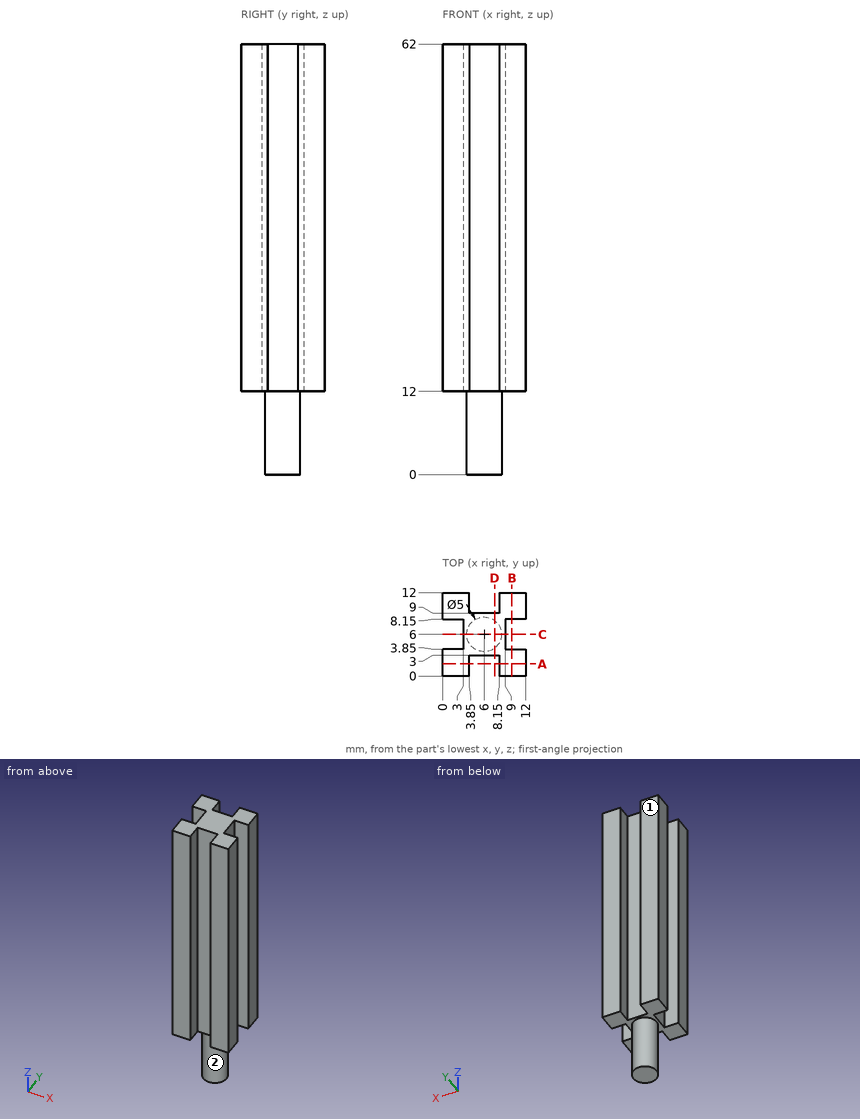
Check sheet for the drawn part. Datum: minimum x, y, z corner. Units: mm. A direction names the side the tool comes from. Round coordinates to 2 decimals unless told otherwise and drop trailing zeros. Order: outer loops, then holes, each group sorted by start corner. A loop starts at its lowest first (then second) coordinate and runs counter-clockwise, first axis right, second up. Notation, with made-up numbers: M 78,-36.75 L 100,-36.75 A20 ccw 100,-21.75 Z; hole C -19.75,9.25 d9. An arc over 180 degrees is marked long. Answer in a Markdown table with one row per item.
(1) Section check D-D on x = 7.5. Record the boundary of the cut face in (y, z), plus the area to 3 significant figures.
Findings:
| item | result |
|---|---|
| outline | M 3,12 L 4,12 L 4,0 L 8,0 L 8,12 L 9,12 L 9,62 L 3,62 Z |
| area | 348 mm^2 |
(2) Material ranges on line 1 along X through (y, z) = (9.75, 57); line 2 along Z through (x, y) = (3.5, 8), recorded low to high. Write a range as from..to.
Findings:
| item | result |
|---|---|
| line 1 | x = 0..3.85, 8.15..12 |
| line 2 | z = 12..62 |
(3) Gauge pin test, flat ends, axial feed: pin 1 (1.3 mm diameter, centred on y = 6, z = 44.5, fed in from -X); pin 2 (1 mm diameter, centred on x = 7, z = 6.5, fed in from +Y); pin 3 (2 mm diameter, centred on x = 5, z = 45.5, fed in from -Y). Record the tip position at first contact, or that the pin passes through.
Findings:
| item | result |
|---|---|
| pin 1 | stops at x = 3 |
| pin 2 | stops at y = 8.45 |
| pin 3 | stops at y = 3 |
(4) Set-up check for the marked faces 1 and 2: record each of +Z, -Z, +X, -X, +Y, -Y from which the full face is reachable in a straight line by a thin tool's end or side.
Findings:
| item | result |
|---|---|
| face 1 | +Z, -Z, +X, -X, +Y |
| face 2 | -Z |
(5) Section check A-A on y = 1.75. Record the boundary of the cut face in (x, z), plus the area to 3 significant figures.
Findings:
| item | result |
|---|---|
| outline | M 0,12 L 3.85,12 L 3.85,62 L 0,62 Z; M 8.15,12 L 12,12 L 12,62 L 8.15,62 Z |
| area | 385 mm^2 |
(6) Section check C-C on y = 6. Record the boundary of the cut face in (x, z).
Findings:
| item | result |
|---|---|
| outline | M 3,12 L 3.5,12 L 3.5,0 L 8.5,0 L 8.5,12 L 9,12 L 9,62 L 3,62 Z |
